Part print with two shaded views. Sizes in mm from the minimum x, y, z corner. A direction names the side the tool comes from. Round coordinates to 2 decimals unless told otherwise and drop trailing zeros. Write each loop counter-clockwise with the first axis right and the second up, starting at its lowest first coordinate (ties: lowest second). Pieces come first, ordered by that corner, then holes.
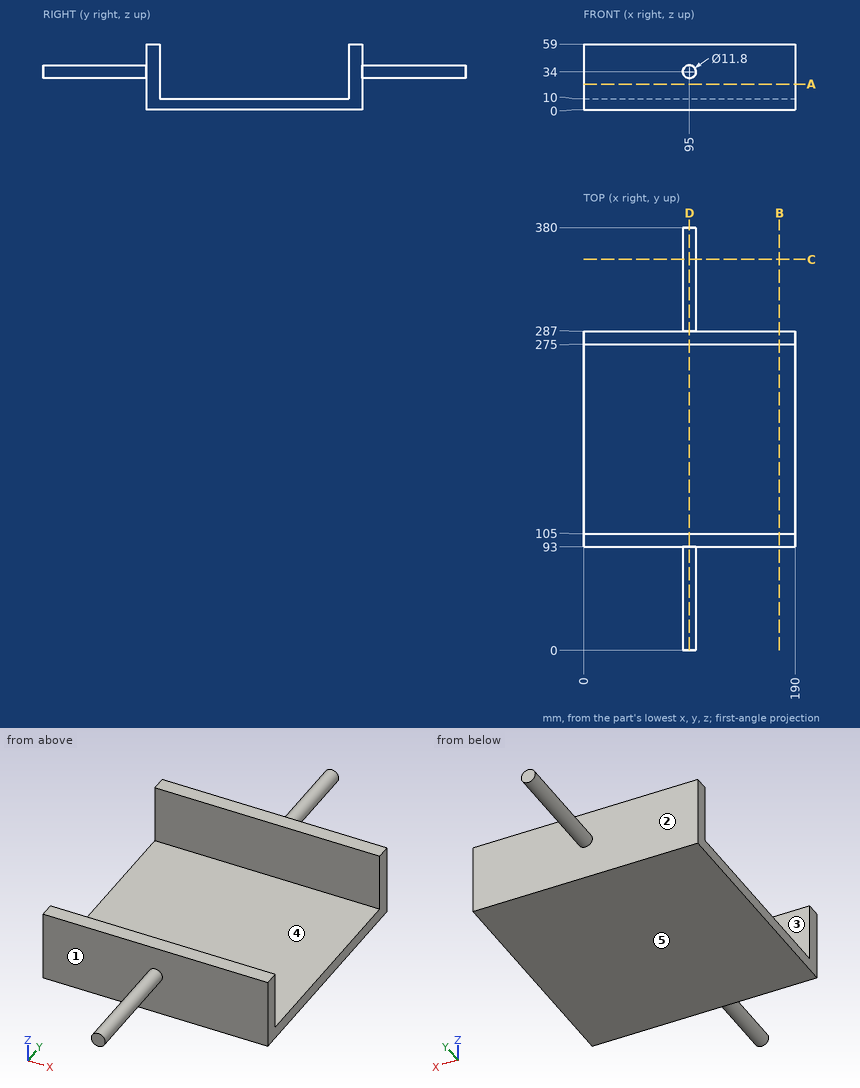
Q1. Cut at C-C on y = 351.5. Write the cut outline in (x, z), plus the area to 3 significant figures.
Values follow:
outline: circle Ø11.8 at (95, 34)
area: 109 mm2
Q2. Drop flat-ended pins along their axis: pin 1 (6 mm diameter, centred on x = 85.5, z = 12, fed in from +Y); pin 2 (8 mm diameter, centred on x = 159.5, z = 41.5, fed in from -Y); pin 3 (6 mm diameter, centred on x = 137, y = 110.5, fed in from +Z). Give the stop position or say it passes through.
Values follow:
pin 1: stops at y = 287
pin 2: stops at y = 93
pin 3: stops at z = 10
Q3. Which spindle directions (+Z, -Z, +X, -X, +Y, -Y) get a long thin tool onto all of the face, cutting with end or side? Do the marked faces 4 and 5. Say none if no direction does.
Values follow:
face 4: +Z, +X, -X
face 5: -Z, +X, -X, +Y, -Y
Q4. Cut at B-B on x = 176. Write the cut outline in (y, z).
Values follow:
outline: (93, 0) - (287, 0) - (287, 59) - (275, 59) - (275, 10) - (105, 10) - (105, 59) - (93, 59) - close
Q5. Wall check: L1, parallel to Y at x = 89.5, z = 52; L2, parallel to Z at x = 176, y = 217.5; L3, parallel to Y at x = 118.5, z = 3.5. Give the ranges that are in metal, low to high.
Values follow:
L1: y = 93 to 105, 275 to 287
L2: z = 0 to 10
L3: y = 93 to 287
Q6. Mould opens along Y. For the marked faces 1, 2 and 3 say: +Y half, -Y half, draft (parallel to the pull), parting line (faces both ways), or undercut.
Values follow:
face 1: -Y half
face 2: +Y half
face 3: undercut
Q7. Cut at D-D on x = 95. Write the cut outline in (y, z), plus the area to 3 significant figures.
Values follow:
outline: (0, 28.1) - (93, 28.1) - (93, 0) - (287, 0) - (287, 28.1) - (380, 28.1) - (380, 39.9) - (287, 39.9) - (287, 59) - (275, 59) - (275, 10) - (105, 10) - (105, 59) - (93, 59) - (93, 39.9) - (0, 39.9) - close
area: 5,310 mm2
Q8. Cut at A-A on z = 23. Write the cut outline in (x, y), plus the area to 3 significant figures.
Values follow:
outline: (0, 93) - (190, 93) - (190, 105) - (0, 105) - close; (0, 275) - (190, 275) - (190, 287) - (0, 287) - close
area: 4,560 mm2
